Autodesk Inventor part; units mm, degrees
ref_plane "YZ Plane" through (0, 0, 0) normal (1, 0, 0) x (0, 1, 0)
ref_plane "XZ Plane" through (0, 0, 0) normal (0, 1, 0) x (-1, 0, 0)
ref_plane "XY Plane" through (0, 0, 0) normal (0, 0, 1) x (1, 0, 0)
sketch "草圖1" plane through (0, 0, 0) normal (0, 0, 1) x (1, 0, 0)
  line L0 (0, 10) -> (20, 10)
  line L1 (20, 10) -> (20, 0)
  line L2 (20, 0) -> (0, 0)
  line L3 (0, 0) -> (0, 10)
  dimension "d0" = 10
  dimension "d1" = 20
extrude "擠出1" add sketch "草圖1" along normal blind 3
sketch "草圖2" plane through (0, 0, 3) normal (0, 0, 1) x (1, 0, 0)
  line L0 (20, 10) -> (0, 10)
  line L1 (20, 0) -> (20, 10)
  line L2 (0, 10) -> (20, 10)
  line L3 (20, 10) -> (20, 8)
  line L4 (20, 8) -> (0, 8)
  line L5 (0, 8) -> (0, 10)
  line L6 (20, 0) -> (0, 0)
  line L7 (0, 0) -> (0, 2)
  line L8 (0, 2) -> (20, 2)
  line L9 (20, 2) -> (20, 0)
  point P0 (0, 0)
  dimension "d4" = 2
  dimension "d5" = 2
extrude "擠出2" add sketch "草圖2" along normal blind 3
CAD build for the part. Positions are in the model's coordinates, mm. A direction names the side the tool comes from. Round coordinates to 2 decimals unless told otherwise and drop trailing zeros. Write each loop counter-clockwise with the first axis right and the second up, starting at its lowest first coordinate (ties: lowest second). Pieces come first, ordered by that corner, then holes. Notation, with made-up numbers: (19, 54) - (72, 54) arc R24 ccw to (72, 70) - close; hole circle Ø6 at (56.25, 32.25). An arc over 180 degrees is marked (long way). Return JSON: item names as keys, results as strings. Group by question number.
Item 1: Band-saw the part on B-B on x = 16. List the corners of the cut face in (y, z), plus the area to 3 significant figures.
Item 2: Band-saw the part on A-A on z = 4.6. List the corners of the cut face in (x, y).
Item 3: Mould opens along Y. For faces 1 (the face through (10, 2, 4)), 2 (the face through (10, 9, 6)), 3 (the face through (10, 0, 3)) say: +Y half, -Y half, draft (parallel to the pull), parting line (faces both ways), or undercut.
Item 4: 3-axis set-ups, long thin cutter, end or side, ignore diameter. For faces 4 (the face through (10, 10, 3)), 5 (the face through (10, 8, 4)): which of +Z, -Z, +X, -X, +Y, -Y reach the whole face in a straight line?
Item 5: Probe probe 1 along Y at (x, z) = (17, 3.5); probe 2 along Z at (x, y) = (3, 3.25). List the from-to ranges inside material, lowest first.
Item 6: Flat gauge pins, fed straight in: pin 1 Ø6 at (x, y) = (10, 3.5) entering from -Z; pin 2 Ø1 at (x, y) = (5.5, 7) entering from +Z. Where does each tip first touch, or does it go through?
Item 7: Band-saw the part on C-C on y = 6. List the corners of the cut face in (x, z), plus the area to 3 significant figures.
Resolved:
{
 "1": {"outline": "(0, 0) - (10, 0) - (10, 6) - (8, 6) - (8, 3) - (2, 3) - (2, 6) - (0, 6) - close", "area": "42.0 mm²"},
 "2": {"outline": "(0, 0) - (20, 0) - (20, 2) - (0, 2) - close; (0, 8) - (20, 8) - (20, 10) - (0, 10) - close"},
 "3": {"face 1": "undercut", "face 2": "draft", "face 3": "-Y half"},
 "4": {"face 4": "+Z, -Z, +X, -X, +Y", "face 5": "+Z, +X, -X"},
 "5": {"probe 1": "y = 0 to 2, 8 to 10", "probe 2": "z = 0 to 3"},
 "6": {"pin 1": "stops at z = 0", "pin 2": "stops at z = 3"},
 "7": {"outline": "(0, 0) - (20, 0) - (20, 3) - (0, 3) - close", "area": "60.0 mm²"}
}
